The listing builds one solid part. Answer for the finished solid, in the listing's coordinates (mm). A direction names the side the tool comes from. Give positions to 0.01 mm unless a question says otherwise; leave off trailing zeros. Loops run counter-clockwise (first coordinate to the right, second up) from the corner with the lowest first, then second, coordinate; pieces in that order, holes last.
Item 1: Section D-D, the plane x = 6.5 is taken. Give the vertices of the cut face in (y, z), and give its area (3 significant figures).
Item 2: Each of these flat-tipped pins is pushed along its axis until it touches: pin 1 Ø8 at (y, z) = (12.5, 44) entering from +X; pin 2 Ø8.5 at (x, y) = (-48, 10) entering from -Z; pin 3 Ø3 at (y, z) = (19.5, 46.5) entering from -X. Where does it stop, or does it pass through?
Item 3: A tool of negligible diameter and unlimited length cuts with its end or side. For faces 1 (the face through (-77.5, 14.2, 45.1)), 2 (the face through (-55, 28, 42)), 3 (the face through (-55, 15, 40)), 4 (the face through (-30, 15, 45)), from which of +Z, -Z, +X, -X, +Y, -Y can it reach the whole face along a straight path? Write none if from no direction.
Item 4: Consider line 1 along Z through (x, y) = (-35.5, 18.25); line 2 along Y through (x, z) = (-33.5, -28.5); line 3 along Z through (x, y) = (-34, 12.5). Determine where each line is inside the solid, lowest interval first.
Item 5: Section B-B, the plane x = -60 is taken. Give the vertices of the cut face in (y, z), and give its area (3 significant figures).
Item 6: Section C-C, the plane y = 16 is taken. Give the vertices of the cut face in (x, z).
Item 7: The mould has two halves that part along X. Classify faces 5 (the face through (-38, 10, 50)), 6 (the face through (-32.5, 14.2, 44.9)), 7 (the face through (-80, 15, 45)): pulls with the +X half, pulls with the -X half, needs draft (parallel to the pull), parting line crosses it, or undercut.
Item 8: Section A-A, the plane z = 45 is taken. Give the vertices of the cut face in (x, y).
from build123d import *

# Parameters (mm, degrees)
SKETCH1_W           = 200
SKETCH1_H           = 100
BOSS_EXTRUDE1_DEPTH = 3
SKETCH2_W           = 50
SKETCH2_H           = 10
BOSS_EXTRUDE2_DEPTH = 25
CUT_EXTRUDE1_DEPTH  = 29


with BuildPart() as part:
    # Sketch1 → Boss-Extrude1 (new body)
    with BuildSketch(Plane(origin=(0, 0, 0), x_dir=(1, 0, 0), z_dir=(0, 1, 0))):
        Rectangle(SKETCH1_W, SKETCH1_H)
    extrude(amount=BOSS_EXTRUDE1_DEPTH)

    # Sketch2 → Boss-Extrude2 (add)
    with BuildSketch(Plane(origin=(0, 3, 0), x_dir=(1, 0, 0), z_dir=(0, 1, 0))):
        with Locations((-55, -45)):
            Rectangle(SKETCH2_W, SKETCH2_H)
    extrude(amount=BOSS_EXTRUDE2_DEPTH)

    # Sketch3 → Cut-Extrude1 (cut, through all)
    with BuildSketch(Plane(origin=(0, 28, 0), x_dir=(1, 0, 0), z_dir=(0, 1, 0))):
        with BuildLine():
            Line((-75, -42.5), (-35, -42.5))
            ThreePointArc((-35, -42.5), (-32.5, -45), (-35, -47.5))
            Line((-35, -47.5), (-75, -47.5))
            ThreePointArc((-75, -47.5), (-77.5, -45), (-75, -42.5))
        make_face()
    extrude(amount=-CUT_EXTRUDE1_DEPTH, mode=Mode.SUBTRACT)


solid = part.part
Worked answers:
1. outline: (0, -50) - (3, -50) - (3, 50) - (0, 50) - close
1. area: 300 mm2
2. pin 1: stops at x = -30
2. pin 2: stops at z = 40
2. pin 3: stops at x = -80
3. face 1: +Y, -Y
3. face 2: +Z, -Z, +X, -X, +Y
3. face 3: -Z, +X, -X, +Y
3. face 4: +Z, -Z, +X, +Y
4. line 1: z = 40 to 42.5, 47.5 to 50
4. line 2: y = 0 to 3
4. line 3: z = 40 to 42.71, 47.29 to 50
5. outline: (0, -50) - (3, -50) - (3, 40) - (28, 40) - (28, 42.5) - (0, 42.5) - close; (0, 47.5) - (28, 47.5) - (28, 50) - (0, 50) - close
5. area: 410 mm2
6. outline: (-80, 40) - (-30, 40) - (-30, 50) - (-80, 50) - close; hole (-75, 42.5) - (-35, 42.5) arc R2.5 ccw to (-35, 47.5) - (-75, 47.5) arc R2.5 ccw to start
7. face 5: needs draft
7. face 6: undercut
7. face 7: pulls with the -X half
8. outline: (-100, 0) - (-77.5, 0) - (-77.5, 28) - (-80, 28) - (-80, 3) - (-100, 3) - close; (-32.5, 0) - (100, 0) - (100, 3) - (-30, 3) - (-30, 28) - (-32.5, 28) - close
